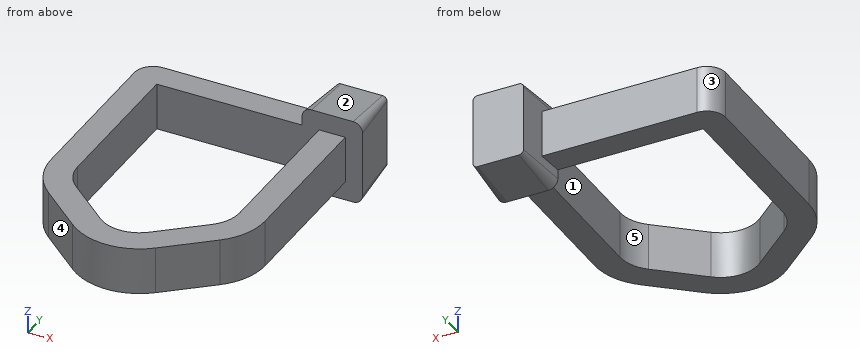
Autodesk Inventor part; units mm, degrees
ref_plane "YZ Plane" through (0, 0, 0) normal (1, 0, 0) x (0, 1, 0)
ref_plane "XZ Plane" through (0, 0, 0) normal (0, 1, 0) x (-1, 0, 0)
ref_plane "XY Plane" through (0, 0, 0) normal (0, 0, 1) x (1, 0, 0)
sketch "Sketch1" plane through (0, 0, 0) normal (0, 0, 1) x (1, 0, 0)
  line L0 (-0.1, 3.0255) -> (8.5, 3.0255)
  line L1 (8.5, 3.0255) -> (8.5, -5.0485)
  line L2 (-0.1, -5.0485) -> (-0.1, 3.0255)
  arc A0 (2.9061, -8.525) -> (5.4939, -8.525) centre (4.2, -7) ccw
  line L3 (0.6061, -6.5735) -> (2.9061, -8.525)
  line L4 (7.7939, -6.5735) -> (5.4939, -8.525)
  arc A1 (-0.1, -5.0485) -> (0.6061, -6.5735) centre (1.9, -5.0485) ccw
  arc A2 (8.7584, -7.5913) -> (9.8881, -5.1512) centre (6.6881, -5.1512) ccw
  line L5 (8.7584, -7.5913) -> (6.3997, -9.5925)
  arc A3 (2.0003, -9.5925) -> (6.3997, -9.5925) centre (4.2, -7) ccw
  line L6 (2.0003, -9.5925) -> (-0.2997, -7.6411)
  arc A4 (-1.5, -5.0485) -> (-0.2997, -7.6411) centre (1.9, -5.0485) ccw
  line L7 (-1.5, -5.0485) -> (-1.5, 3.4255)
  line L8 (-0.5, 4.4255) -> (9.8881, 4.4255)
  line L9 (9.8881, 4.4255) -> (9.8881, -5.1512)
  arc A5 (-0.5, 4.4255) -> (-1.5, 3.4255) centre (-0.5, 3.4255) ccw
  arc A6 (7.7939, -6.5735) -> (8.5, -5.0485) centre (6.5, -5.0485) ccw
  point P0 (-0.1, -5.9745)
  dimension "d1" = 9
  dimension "d2" = 4
  dimension "d4" = 2
  dimension "d5" = 1.4
  dimension "d6" = 1
  dimension "d16" = 2
  dimension "d19" = 8.6
  dimension "d20" = 2.3
extrude "Extrusion1" add sketch "Sketch1" along normal blind 2.5
sketch "Sketch2" plane through (-0.1, 3.0255, 2.5) normal (0, -1, 0) x (1, 0, 0)
  line L0 (8.2, 1) -> (10.4, 1)
  line L1 (10.9, 0.5) -> (10.9, -3)
  line L2 (10.4, -3.5) -> (8.2, -3.5)
  line L3 (7.7, -3) -> (7.7, 0.5)
  arc A0 (8.2, 1) -> (7.7, 0.5) centre (8.2, 0.5) ccw
  arc A1 (10.9, 0.5) -> (10.4, 1) centre (10.4, 0.5) ccw
  arc A2 (10.4, -3.5) -> (10.9, -3) centre (10.4, -3) ccw
  arc A3 (7.7, -3) -> (8.2, -3.5) centre (8.2, -3) ccw
  line L4 (-1.4, -2.5) -> (-1.4, 0)
  point P0 (7.7, 1)
  point P1 (10.9, -3.5)
  point P2 (10.9, 1)
  dimension "d9" = 4.5
  dimension "d10" = 3.2
  dimension "d13" = 0.5
  dimension "d21" = 9.1
extrude "Extrusion2" add sketch "Sketch2" against normal blind 3 draft -5
properties part number "fastener_02"
The model under review builds one solid part; all positions refer to its coordinate system, in mm. Face numbers are marked on the shaded views. A direction names the side the tool comes from. Round coordinates to 2 decimals unless told otherwise and drop trailing zeros. Order: outer loops, then holes, each group sorted by start corner. A loop starts at its lowest first (then second) coordinate and runs counter-clockwise, first axis right, second up. Notation, with made-up numbers: (11.5, -35.5) -> (33.5, -35.5) arc R17 cw to (33.5, -8.5) -> close; hole circle Ø8 at (10, -7.5). An arc over 180 degrees is marked (long way). Use a Markdown table: item, result.
Q1. Mouldability with a two-part tool opening along X and no side actions: class the marked faces 1, 2 and 3 as +X half, -X half, draft (parallel to the pull), parting line (faces both ways), or undercut.
Values:
| item | result |
|---|---|
| face 1 | undercut |
| face 2 | draft |
| face 3 | -X half |
Q2. We need section C-C on x = 6. Write out the cut boundary in (y, z), then the cut area to 3 significant figures.
Values:
| item | result |
|---|---|
| outline | (-9.88, 0) -> (-8.1, 0) -> (-8.1, 2.5) -> (-9.88, 2.5) -> close; (3.03, 0) -> (4.43, 0) -> (4.43, 2.5) -> (3.03, 2.5) -> close |
| area | 7.97 mm^2 |
Q3. Clearance check with flat-ended pins moving along their axes: P1, Ø1.5, axis at y = -6, z = 2, coming from the -X side; P2, Ø1.2, axis at y = -1.5, z = 1.5, coming from the +X side; P3, Ø1, axis at x = 6, z = 1, coming from the +Y side. State where each tip first meets the part, or that it passes through.
Values:
| item | result |
|---|---|
| P1 | stops at x = -1.49 |
| P2 | stops at x = 9.89 |
| P3 | stops at y = 4.43 |
Q4. We need section D-D on x = 9.5. Write out the cut boundary in (y, z), then the cut area to 3 significant figures.
Values:
| item | result |
|---|---|
| outline | (-6.68, 0) -> (3.03, 0) -> (3.03, -1) -> (6.03, -0.74) -> (6.03, 3.24) -> (3.03, 3.5) -> (3.03, 2.5) -> (-6.68, 2.5) -> close |
| area | 37.0 mm^2 |
Q5. We need section B-B on y = -3.25. Write out the cut boundary in (x, z).
Values:
| item | result |
|---|---|
| outline | (-1.5, 0) -> (-0.1, 0) -> (-0.1, 2.5) -> (-1.5, 2.5) -> close; (8.5, 0) -> (9.89, 0) -> (9.89, 2.5) -> (8.5, 2.5) -> close |
Q6. We need section A-A on z = 0.3. Write out the cut boundary in (x, y) (1 decimal).
Values:
| item | result |
|---|---|
| outline | (-1.5, -5) arc R3.4 ccw to (-0.3, -7.6) -> (2, -9.6) arc R3.4 ccw to (6.4, -9.6) -> (8.8, -7.6) arc R3.2 ccw to (9.9, -5.2) -> (9.9, 3) -> (10.8, 3) -> (10.5, 6) -> (7.9, 6) -> (7.7, 4.4) -> (-0.5, 4.4) arc R1 ccw to (-1.5, 3.4) -> close; hole (-0.1, -5) arc R2 ccw to (0.6, -6.6) -> (2.9, -8.5) arc R2 ccw to (5.5, -8.5) -> (7.8, -6.6) arc R2 ccw to (8.5, -5) -> (8.5, 3) -> (-0.1, 3) -> close |
Q7. For line 1 (Y direction, x = 10, z = 3); line 2 (X direction, y = -3.25, z = 1.2); line 3 (Z direction, x = 1.25, y = -8.25), list the stretches that pass through material, from the lowest coordinate up.
Values:
| item | result |
|---|---|
| line 1 | y = 3.03 to 6.03 |
| line 2 | x = -1.5 to -0.1, 8.5 to 9.89 |
| line 3 | z = 0 to 2.5 |
Q8. Tool access review of the marked faces 4 and 5: name each direction out of +Z, -Z, +X, -X, +Y, -Y from which nothing blocks a thin tool from reaching the whole face with its end or side.
Values:
| item | result |
|---|---|
| face 4 | +Z, -Z, -X, -Y |
| face 5 | +Z, -Z |
